```python
from build123d import *

# Parameters (mm, degrees)
SKETCH1_W           = 25
SKETCH1_H           = 25
BOSS_EXTRUDE1_DEPTH = 25
CUT_EXTRUDE1_DEPTH  = 26


with BuildPart() as part:
    # Sketch1 → Boss-Extrude1 (new body)
    with BuildSketch(Plane(origin=(0, 0, 0), x_dir=(1, 0, 0), z_dir=(0, 1, 0))):
        Rectangle(SKETCH1_W, SKETCH1_H)
    extrude(amount=BOSS_EXTRUDE1_DEPTH)

    # Sketch2 → Cut-Extrude1 (cut, through all)
    with BuildSketch(Plane.XY.offset(12.5)):
        with BuildLine():
            Line((-2.179449472, 17), (0, 19.179449472))
            Line((0, 19.179449472), (2.179449472, 17))
            ThreePointArc((2.179449472, 17), (0, 7.5), (-2.179449472, 17))
        make_face()
    extrude(amount=-CUT_EXTRUDE1_DEPTH, mode=Mode.SUBTRACT)


solid = part.part
```
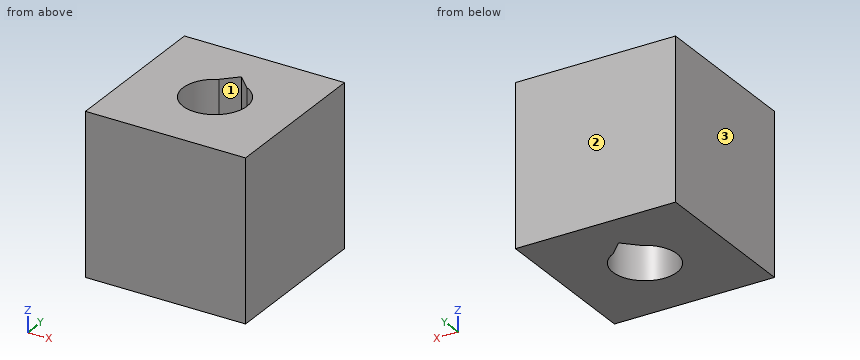
Part model, mm, in its own coordinate system. Face numbers are marked on the shaded views. Round coordinates to 2 decimals unless told otherwise and drop trailing zeros. Loops run counter-clockwise (first coordinate to the right, second up) from the corner with the lowest first, then second, coordinate; pieces in that order, holes last.
Item 1: Cut at A-A, the plane y = 12.5. Give the cut face in (x, z).
Item 2: Drill centre lines: line 1 (X direction, y = 12.5, z = 0.5); line 2 (X direction, y = 9, z = -0.75); line 3 (Y direction, x = -4.5, z = 3). Where is each one in solid material? Low to high.
Item 3: Mould opens along Y. For the marked faces 1, 2 and 3 say: +Y half, -Y half, draft (parallel to the pull), parting line (faces both ways), or undercut.
Item 4: Cut at C-C, the plane z = 6. Give the cut face in (x, y), then the cut area to 3 significant figures.
Item 5: Cut at B-B, the plane x = -0.5. Give the cut face in (y, z), then the cut area to 3 significant figures.
A:
1. outline: (-12.5, -12.5) - (-5, -12.5) - (-5, 12.5) - (-12.5, 12.5) - close; (5, -12.5) - (12.5, -12.5) - (12.5, 12.5) - (5, 12.5) - close
2. line 1: x = -12.5 to -5, 5 to 12.5
2. line 2: x = -12.5 to -3.57, 3.57 to 12.5
2. line 3: y = 0 to 10.32, 14.68 to 25
3. face 1: undercut
3. face 2: +Y half
3. face 3: draft
4. outline: (-12.5, 0) - (12.5, 0) - (12.5, 25) - (-12.5, 25) - close; hole (-2.18, 17) arc R5 ccw (long way) to (2.18, 17) - (0, 19.18) - close
4. area: 543 mm2
5. outline: (0, -12.5) - (7.53, -12.5) - (7.53, 12.5) - (0, 12.5) - close; (18.68, -12.5) - (25, -12.5) - (25, 12.5) - (18.68, 12.5) - close
5. area: 346 mm2
